Drawing for the job (mm, zero at the part's lowest x, y, z). Give positions to 0.01 mm unless a question says otherwise; leave off trailing zeros. Loops run counter-clockwise (first coordinate to the right, second up) from the corner with the lowest first, then second, coordinate; pieces in that order, holes last. Notation, with made-up numbers: (30, 65.5) -> (63, 65.5) arc R17 cw to (63, 88.5) -> close; hole circle Ø2 at (-9.75, 60.5). An arc over 180 degrees is marked (long way). Answer in a Markdown table with one row per item. Add a question column.
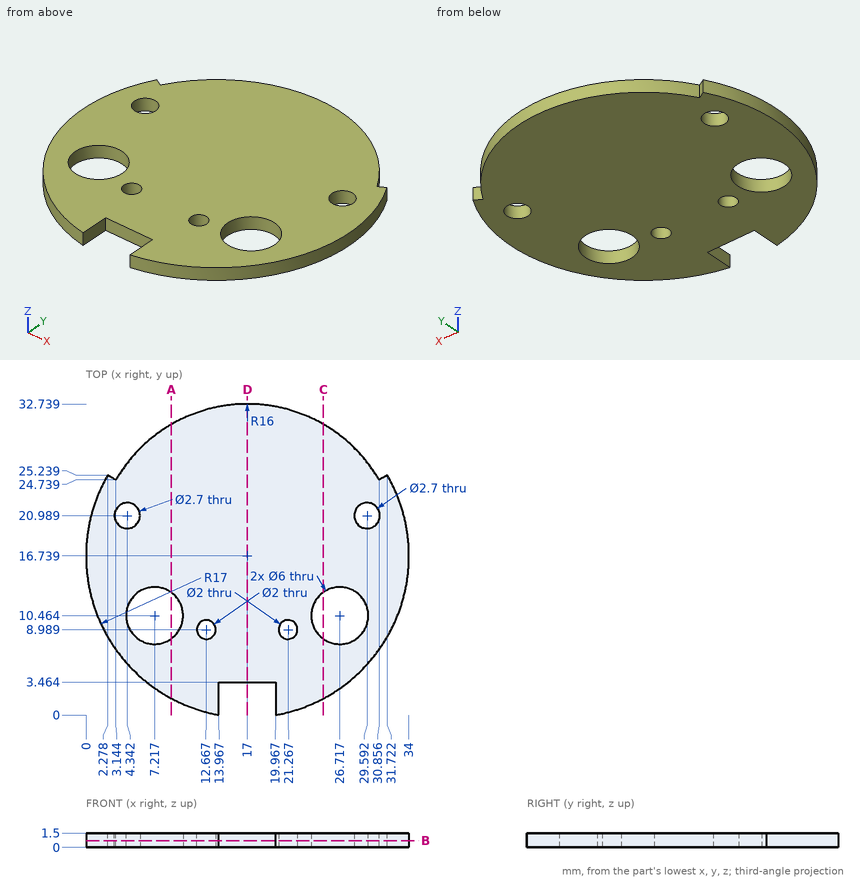
(1) Saw through at B-B, the plane z = 0.7. State how many separate pieces and enclosed holes the cut face has, then the cut area to 3 significant figures.
(2) Saw through at A-A, the plane x = 9. List the corners of the cut face in (y, z) (1 decimal).
(3) Saw through at D-D, the plane x = 17. List the corners of the cut face in (y, z) (1 decimal).
(4) Wall check: line 1 along Y through (x, z) = (21, 1.3) (1 decimal); line 2 along X through (y, z) = (21, 0.65); line 3 along Y through (x, z) = (4, 0.6) (1 decimal). Give the ranges that are in metal, low to high. Write a range as from..to.
(5) Saw through at C-C, the plane x = 25. List the corners of the cut face in (y, z) (1 decimal).
(6) Flat gauge pins, fed straight in: pin 1 Ø3 at (x, y) = (21.27, 8.99) entering from -Z; pin 2 Ø2.5 at (x, y) = (4.34, 20.99) entering from -Z. Where does each tip first touch, or does it go through?
Worked answers:
| question | item | result |
|---|---|---|
| 1 | separate pieces | 1 |
| 1 | enclosed holes | 6 |
| 1 | area | 777 mm^2 |
| 2 | outline | (1.7, 0) -> (8.1, 0) -> (8.1, 1.5) -> (1.7, 1.5) -> close; (12.9, 0) -> (30.6, 0) -> (30.6, 1.5) -> (12.9, 1.5) -> close |
| 3 | outline | (3.5, 0) -> (32.7, 0) -> (32.7, 1.5) -> (3.5, 1.5) -> close |
| 4 | line 1 | 0.2..8, 10..32.2 |
| 4 | line 2 | 0.54..2.99, 5.69..28.24, 30.94..33.46 |
| 4 | line 3 | 5.8..19.7, 22.3..26.1 |
| 5 | outline | (1.7, 0) -> (8, 0) -> (8, 1.5) -> (1.7, 1.5) -> close; (12.9, 0) -> (30.6, 0) -> (30.6, 1.5) -> (12.9, 1.5) -> close |
| 6 | pin 1 | z = 0 |
| 6 | pin 2 | through |
